Check sheet for the modelled part. Datum: model origin and axes. Units: mm. A direction names the side the tool comes from. Coordinates: 2 decimals unless noted, no trailing zeros. Order: outer loops, then holes, each group sorted by start corner. A loop starts at its lowest first (then second) coordinate and runs counter-clockwise, first axis right, second up.
from build123d import *

# Parameters (mm, degrees)
F3_DEPTH = 12


with BuildPart() as f1:
    # F0 (on Front) → F1 (revolve)
    with BuildSketch(Plane.XZ):
        Polygon((35, 4), (35, 0), (65, 0), (65, 12), (12.7, 12), (12.7, 6), (11, 6), (11, 4), align=None)
    revolve(axis=Axis((0, 0, 8.603251), (0, 0, 1)))

    # F2 (on face) → F3 (cut)
    with BuildSketch(Plane.XY.offset(12)):
        with BuildLine():
            ThreePointArc((-4.496233, 54.815909), (0, 50.5), (4.496233, 54.815909))
            ThreePointArc((4.496233, 54.815909), (4.499058, 54.907935), (4.5, 55))
            ThreePointArc((4.5, 55), (-0.092065, 59.499058), (-4.496233, 54.815909))
        make_face()
        with BuildLine():
            ThreePointArc((-50.5, 0), (-51.753586, 3.116215), (-54.815909, 4.496233))
            ThreePointArc((-54.815909, 4.496233), (-59.5, 0), (-54.815909, -4.496233))
            ThreePointArc((-54.815909, -4.496233), (-51.753586, -3.116215), (-50.5, 0))
        make_face()
        with BuildLine():
            ThreePointArc((4.5, -55), (4.499058, -54.907935), (4.496233, -54.815909))
            ThreePointArc((4.496233, -54.815909), (0, -50.5), (-4.496233, -54.815909))
            ThreePointArc((-4.496233, -54.815909), (-0.092065, -59.499058), (4.5, -55))
        make_face()
        with BuildLine():
            ThreePointArc((59.5, 0), (58.116215, 3.246414), (54.815909, 4.496233))
            ThreePointArc((54.815909, 4.496233), (50.5, 0), (54.815909, -4.496233))
            ThreePointArc((54.815909, -4.496233), (58.116215, -3.246414), (59.5, 0))
        make_face()
    extrude(amount=-F3_DEPTH, mode=Mode.SUBTRACT)


solid = f1.part
(1) Cross-section at C-C (y = 52). Enter the section's corners in (x, z), and give its area (4 significant figures).
Filled in:
outline: (-39, 0) - (-3.35, 0) - (-3.35, 12) - (-39, 12) - close; (3.35, 0) - (39, 0) - (39, 12) - (3.35, 12) - close
area: 855.5 mm2
(2) Go/stop test with flat-tipped pins: P1, Ø2, axis at x = 24.5, y = 20, coming from the -Z side; P2, Ø3, axis at y = 21.5, z = 10.5, coming from the +X side; P3, Ø7.5, axis at x = -2.5, y = 4.5, coming from the +Z side; P4, Ø5, axis at x = -36, z = 6, coming from the -Y side. Record where each tip stops, or that it passes through.
Filled in:
P1: stops at z = 4
P2: stops at x = 61.85
P3: passes through
P4: stops at y = -55.7
(3) Release check for a two-part mould opening along Y. For faces 4 (the cylindrical face through (62, 19.52, 6.08)), 5 (the cylindrical face through (-2.38, -10.74, 4.99)), 6 (the flat face through (14, 1, 12)) record: +Y half, -Y half, draft (parallel to the pull), parting line (faces both ways), or undercut.
Filled in:
face 4: parting line
face 5: undercut
face 6: draft
(4) Cross-section at D-D (x = 20). Enter the section's corners in (y, z), and give its area (3 significant figures).
Filled in:
outline: (-61.85, 0) - (-28.72, 0) - (-28.72, 4) - (28.72, 4) - (28.72, 0) - (61.85, 0) - (61.85, 12) - (-61.85, 12) - close
area: 1,250 mm2
(5) Thickness scan on probe 1 along Z at (x, y) = (-12, -27.5); probe 2 along Y at (x, z) = (-51.5, 10.75); probe 3 along Y at (x, z) = (10, 5). Record the ranges inside material, lowest first.
Filled in:
probe 1: z = 4 to 12
probe 2: y = -39.66 to -2.83, 2.83 to 39.66
probe 3: y = -64.23 to -4.58, 4.58 to 64.23
(6) Tool access check on faces 1 (the flat face through (-0.1, 11.3, 6)), 2 (the flat face through (-28, -28, 0)), 3 (the cylindrical face through (-28, -21, 2)). Record the directions out of +Z, -Z, +X, -X, +Y, -Y that give a thin tool (end or side, any length) a straight path to the whole face; none if there is none.
Filled in:
face 1: +Z
face 2: -Z, +X, -X, +Y, -Y
face 3: -Z
(7) Cross-section at B-B (z = 10.5). Enter the section's corners in (x, y).
Filled in:
outline: circle Ø130 at (0, 0); hole circle Ø9 at (-55, 0); hole circle Ø25.4 at (0, 0); hole (4.5, -55) arc R4.5 ccw to (4.5, -54.82) arc R4.5 ccw (long way) to start; hole (4.5, 54.82) arc R4.5 ccw to (4.5, 55) arc R4.5 ccw (long way) to start; hole circle Ø9 at (55, 0)
(8) Cross-section at A-A (x = 0). Enter the section's corners in (y, z).
Filled in:
outline: (-65, 0) - (-59.5, 0) - (-59.5, 12) - (-65, 12) - close; (-50.5, 0) - (-35, 0) - (-35, 4) - (-11, 4) - (-11, 6) - (-12.7, 6) - (-12.7, 12) - (-50.5, 12) - close; (11, 4) - (35, 4) - (35, 0) - (50.5, 0) - (50.5, 12) - (12.7, 12) - (12.7, 6) - (11, 6) - close; (59.5, 0) - (65, 0) - (65, 12) - (59.5, 12) - close
